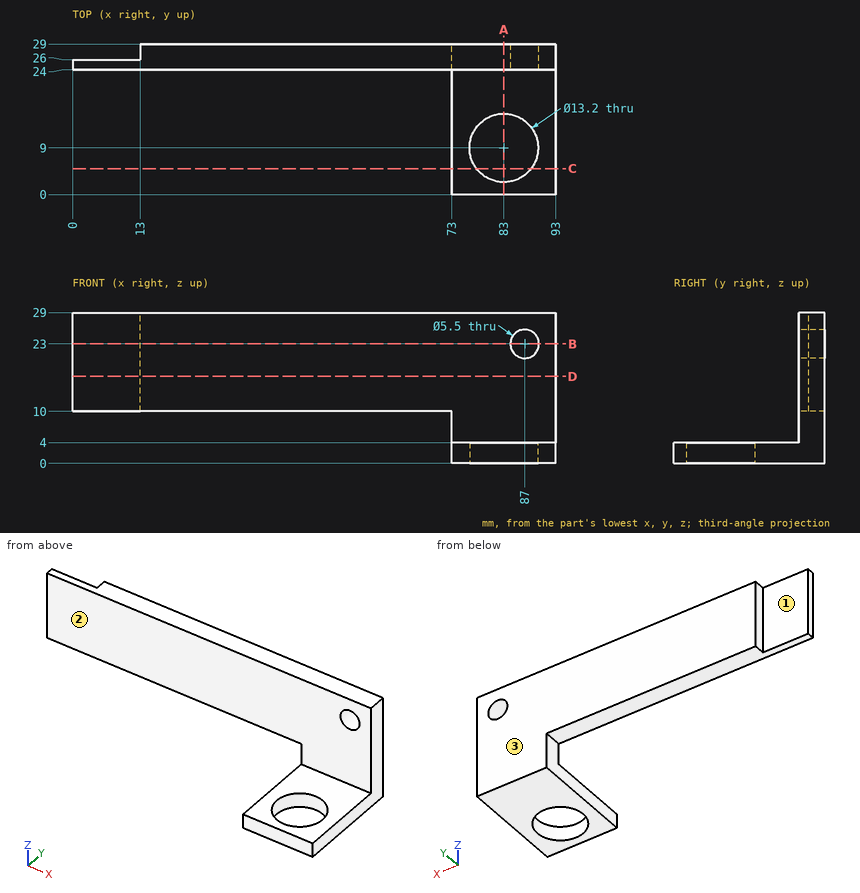
Source: three-view drawing plus pictorial views. Frame: mm from the lowest corner of the part. A direction names the side the tool comes from. Round coordinates to 2 decimals unless told otherwise and drop trailing zeros. Loops run counter-clockwise (first coordinate to the right, second up) from the corner with the lowest first, then second, coordinate; pieces in that order, holes last. Notation, with made-up numbers: (11, 46) -> (35, 46) arc R20 ccw to (35, 66) -> close; hole circle Ø3 at (-17, -36.75). An arc over 180 degrees is marked (long way). Use one line per item in the form item = value.
Item 1: Access query for the marked faces 1, 2 and 3. Directions: +Z, -Z, +X, -X, +Y, -Y. A direction counts if a zero-diameter tool reaches every point of the face in a straight line with its end or side. Return the directions, or none.
Evaluation:
face_1 = +Z, -Z, -X, +Y
face_2 = +Z, +X, -X, -Y
face_3 = +Z, -Z, +X, -X, +Y
Item 2: Cut plane A-A on x = 83. Output: boundary loops of the cut face in (y, z), then the cut area to 3 significant figures.
Evaluation:
outline = (0, 0) -> (2.4, 0) -> (2.4, 4) -> (0, 4) -> close; (15.6, 0) -> (29, 0) -> (29, 29) -> (24, 29) -> (24, 4) -> (15.6, 4) -> close
area = 188 mm2
Item 3: Contact query for flat-ended pins moving along their axis: pin 1 Ø5.5 at (x, y) = (50.5, 27.5) entering from -Z; pin 2 Ø6 at (x, z) = (30.5, 25) entering from -Y; pin 3 Ø3.5 at (y, z) = (28, 18) entering from -X. Output: stop coordinate, or through.
Evaluation:
pin_1 = 10
pin_2 = 24
pin_3 = 13
Item 4: Cut plane C-C on y = 5. Output: boundary loops of the cut face in (x, z), then the cut area to 3 significant figures.
Evaluation:
outline = (73, 0) -> (77.75, 0) -> (77.75, 4) -> (73, 4) -> close; (88.25, 0) -> (93, 0) -> (93, 4) -> (88.25, 4) -> close
area = 38.0 mm2
Item 5: Cut plane D-D on z = 16.75. Output: boundary loops of the cut face in (x, y), then the cut area to 3 significant figures.
Evaluation:
outline = (0, 24) -> (93, 24) -> (93, 29) -> (13, 29) -> (13, 26) -> (0, 26) -> close
area = 426 mm2
Item 6: Material intervals for probe 1 along Z at (x, y) = (87, 26.65); probe 2 along Y at (x, z) = (87.5, 16); probe 3 along X at (y, z) = (3.25, 3), sorted ascending.
Evaluation:
probe_1 = 0 to 20.25, 25.75 to 29
probe_2 = 24 to 29
probe_3 = 73 to 79.76, 86.24 to 93
Item 7: Cut plane B-B on z = 23. Output: boundary loops of the cut face in (x, y), then the cut area to 4 significant figures.
Evaluation:
outline = (0, 24) -> (84.25, 24) -> (84.25, 29) -> (13, 29) -> (13, 26) -> (0, 26) -> close; (89.75, 24) -> (93, 24) -> (93, 29) -> (89.75, 29) -> close
area = 398.5 mm2
